Read the model definition and answer for the solid it produces. Units are mm, in the model's axes. Give positions to 0.01 mm unless a question says otherwise; leave off trailing zeros. Write each loop counter-clockwise with the first axis right and the second up, starting at its lowest first coordinate (ties: lowest second). Pieces come first, ordered by that corner, then holes. Notation, with made-up numbers: (-33.75, 18.5) - (-11.75, 18.5) arc R16 cw to (-11.75, 24.5) - close; hole circle Ø6 at (-33, -30.75). An arc over 180 degrees is marked (long way). Answer as CSV lines item,"result".
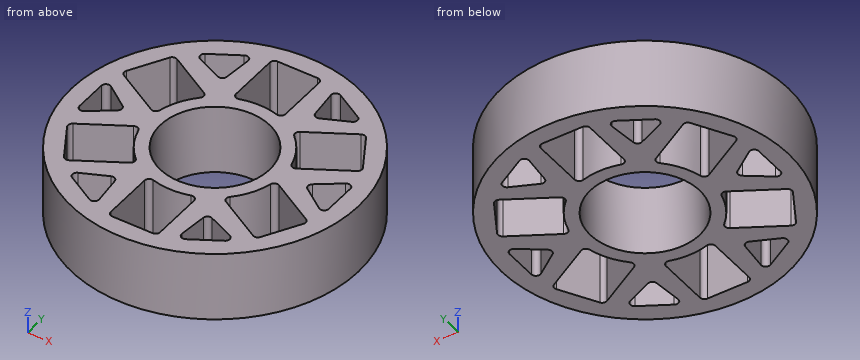
Autodesk Inventor part; units mm, degrees
ref_plane "YZ Plane" through (0, 0, 0) normal (1, 0, 0) x (0, 1, 0)
ref_plane "XZ Plane" through (0, 0, 0) normal (0, 1, 0) x (-1, 0, 0)
ref_plane "XY Plane" through (0, 0, 0) normal (0, 0, 1) x (1, 0, 0)
sketch "Sketch1" plane through (0, 0, 0) normal (0, 0, 1) x (1, 0, 0)
  circle A0 centre (0, 0) radius 19.939
  circle A1 centre (0, 0) radius 52.3875
  line L0 (-9.2075, 22.9897) -> (-9.2075, 45.5957)
  line L1 (-9.2075, 45.5957) -> (8.8265, 45.5957)
  line L2 (8.8265, 45.5957) -> (8.8265, 23.1387)
  line L3 (-44.0908, 14.8239) -> (-35.0738, 30.4418)
  line L4 (-35.0738, 30.4418) -> (-15.6254, 19.2133)
  line L5 (-24.5134, 3.5209) -> (-44.0908, 14.8239)
  line L6 (-34.8833, -30.7718) -> (-43.9003, -15.1539)
  line L7 (-43.9003, -15.1539) -> (-24.4519, -3.9254)
  line L8 (-15.3059, -19.4688) -> (-34.8833, -30.7718)
  line L9 (9.2075, -45.5957) -> (-8.8265, -45.5957)
  line L10 (-8.8265, -45.5957) -> (-8.8265, -23.1387)
  line L11 (9.2075, -22.9897) -> (9.2075, -45.5957)
  line L12 (44.0908, -14.8239) -> (35.0738, -30.4418)
  line L13 (35.0738, -30.4418) -> (15.6254, -19.2133)
  line L14 (24.5134, -3.5209) -> (44.0908, -14.8239)
  line L15 (34.8833, 30.7718) -> (43.9003, 15.1539)
  line L16 (43.9003, 15.1539) -> (24.4519, 3.9254)
  line L17 (15.3059, 19.4688) -> (34.8833, 30.7718)
  arc A2 (8.8265, 23.1387) -> (-9.2075, 22.9897) centre (0, 0) ccw
  arc A3 (-15.6254, 19.2133) -> (-24.5134, 3.5209) centre (0, 0) ccw
  arc A4 (24.4519, 3.9254) -> (15.3059, 19.4688) centre (0, 0) ccw
  arc A5 (15.6254, -19.2133) -> (24.5134, -3.5209) centre (0, 0) ccw
  arc A6 (-24.4519, -3.9254) -> (-15.3059, -19.4688) centre (0, 0) ccw
  arc A7 (-8.8265, -23.1387) -> (9.2075, -22.9897) centre (0, 0) ccw
  line L18 (-45.5802, 9.2075) -> (-32.8802, 0)
  line L19 (-32.8802, 0) -> (-45.5802, -9.2075)
  line L20 (-45.5802, -9.2075) -> (-45.5802, 9.2075)
  line L21 (-30.764, -34.8699) -> (-16.4401, -28.4751)
  line L22 (-14.8162, -44.0774) -> (-30.764, -34.8699)
  line L23 (-16.4401, -28.4751) -> (-14.8162, -44.0774)
  line L24 (14.8162, -44.0774) -> (16.4401, -28.4751)
  line L25 (30.764, -34.8699) -> (14.8162, -44.0774)
  line L26 (16.4401, -28.4751) -> (30.764, -34.8699)
  line L27 (45.5802, -9.2075) -> (32.8802, 0)
  line L28 (45.5802, 9.2075) -> (45.5802, -9.2075)
  line L29 (32.8802, 0) -> (45.5802, 9.2075)
  line L30 (30.764, 34.8699) -> (16.4401, 28.4751)
  line L31 (14.8162, 44.0774) -> (30.764, 34.8699)
  line L32 (16.4401, 28.4751) -> (14.8162, 44.0774)
  line L33 (-14.8162, 44.0774) -> (-16.4401, 28.4751)
  line L34 (-30.764, 34.8699) -> (-14.8162, 44.0774)
  line L35 (-16.4401, 28.4751) -> (-30.764, 34.8699)
  dimension "d0" = 39.878
  dimension "d3" = 104.775
  dimension "d38" = 22.606
  dimension "d39" = 18.034
  dimension "d40" = 9.2075
  dimension "d41" = 360
  dimension "d42" = 9.2075
  dimension "d43" = 9.2075
  dimension "d44" = 9.2075
  dimension "d45" = 12.7
  dimension "d46" = 12.7
  dimension "d49" = 360
extrude "Extrusion2" add sketch "Sketch1" along normal blind 25.4
fillet "Fillet1" radius 1.651 42 edges at (-15.6254, 19.2133, 12.7) (8.8265, 45.5957, 12.7) (30.764, 34.8699, 12.7) (43.9003, 15.1539, 12.7) (-32.8802, 0, 12.7) (-15.3059, -19.4688, 12.7) (-44.0908, 14.8239, 12.7) (-30.764, 34.8699, 12.7) (15.3059, 19.4688, 12.7) (15.6254, -19.2133, 12.7) (32.8802, 0, 12.7) (-30.764, -34.8699, 12.7) (-43.9003, -15.1539, 12.7) (-9.2075, 22.9897, 12.7) (16.4401, 28.4751, 12.7) (24.4519, 3.9254, 12.7) (9.2075, -45.5957, 12.7) (35.0738, -30.4418, 12.7) (45.5802, -9.2075, 12.7) (-14.8162, -44.0774, 12.7) (-24.5134, 3.5209, 12.7) (8.8265, 23.1387, 12.7) (-16.4401, 28.4751, 12.7) (-34.8833, -30.7718, 12.7) (-8.8265, -45.5957, 12.7) (14.8162, -44.0774, 12.7) (-45.5802, -9.2075, 12.7) (-45.5802, 9.2075, 12.7) (-35.0738, 30.4418, 12.7) (-9.2075, 45.5957, 12.7) (-8.8265, -23.1387, 12.7) (24.5134, -3.5209, 12.7) (16.4401, -28.4751, 12.7) (14.8162, 44.0774, 12.7) (9.2075, -22.9897, 12.7) (44.0908, -14.8239, 12.7) (30.764, -34.8699, 12.7) (34.8833, 30.7718, 12.7) (45.5802, 9.2075, 12.7) (-16.4401, -28.4751, 12.7) (-24.4519, -3.9254, 12.7) (-14.8162, 44.0774, 12.7)
properties part number "EXPANDED FLEX WHEEL"
(1) Each of these flat-tipped pins is pushed along its axis until it touches: P1, Ø8, axis at y = 7, z = 13, coming from the -X side; P2, Ø2, axis at x = 3.5, z = 19.5, coming from the -Y side; P3, Ø1.5, axis at x = -18, z = 11, coming from the -Y side; P4, Ø3.5, axis at y = 1.5, z = 10.5, coming from the +X side. Where does it stop, or does it pass through?
Worked out:
P1,"stops at x = -52.3"
P2,"stops at y = -52.33"
P3,"stops at y = -49.47"
P4,"stops at x = 52.39"
(2) A cutting plane is placed at A-A (y = 0). Write down the section's boundary in (x, z), and give its area (3 significant figures).
Worked out:
outline,"(-52.39, 0) - (-45.58, 0) - (-45.58, 25.4) - (-52.39, 25.4) - close; (-34.04, 0) - (-19.94, 0) - (-19.94, 25.4) - (-34.04, 25.4) - close; (19.94, 0) - (34.04, 0) - (34.04, 25.4) - (19.94, 25.4) - close; (45.58, 0) - (52.39, 0) - (52.39, 25.4) - (45.58, 25.4) - close"
area,"1,060 mm^2"
(3) Find the intervals of material crossed by L1, parallel to Y at x = 0, z = 17; L2, parallel to Y at x = 40, z = 18.5; L3, parallel to X at y = 2, z = 10.5, in increasing order.
Worked out:
L1,"y = -52.39 to -45.6, -24.77 to -19.94, 19.94 to 24.77, 45.6 to 52.39"
L2,"y = -33.83 to -21.91, -12.46 to -5.16, 5.16 to 12.9, 21.91 to 33.83"
L3,"x = -52.35 to -45.58, -35.64 to -19.84, 19.84 to 35.64, 45.58 to 52.35"
(4) A cutting plane is placed at B-B (x = 0). Write down the section's boundary in (y, z), and give its area (3 significant figures).
Worked out:
outline,"(-52.39, 0) - (-45.6, 0) - (-45.6, 25.4) - (-52.39, 25.4) - close; (-24.77, 0) - (-19.94, 0) - (-19.94, 25.4) - (-24.77, 25.4) - close; (19.94, 0) - (24.77, 0) - (24.77, 25.4) - (19.94, 25.4) - close; (45.6, 0) - (52.39, 0) - (52.39, 25.4) - (45.6, 25.4) - close"
area,"590 mm^2"
(5) A cutting plane is placed at C-C (z = 13.25). Count the separate pieces of the cut face and the enclosed holes in it, and give its area (3 significant figures).
Worked out:
separate pieces,"1"
enclosed holes,"13"
area,"4,410 mm^2"
